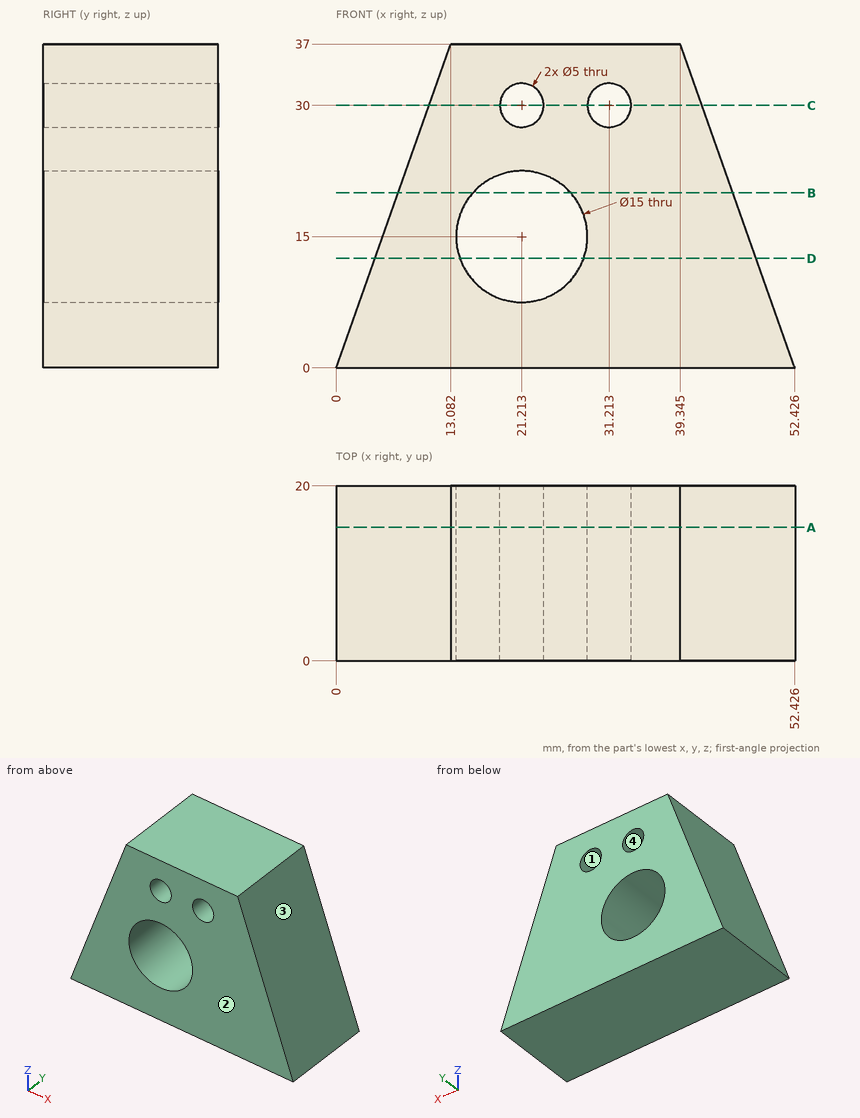
Design review of the part shown in the three views and the two pictorial views. Dimensions are in mm from the part's minimum x, y and z. Give positions to 0.01 mm unless a question says otherwise; leave off trailing zeros. Write each loop counter-clockwise with the first axis right and the second up, starting at its lowest first coordinate (ties: lowest second). Pieces come first, ordered by that corner, then holes. Notation, with made-up numbers: M 11,13 L 68,13 A13 cw 68,24 Z; hole C -25.5,-27.75 d7. An arc over 180 degrees is marked long. Answer in a Markdown table with one row per item.
Item 1: Add section D-D on z = 12.5. Give the boundary of the cut face in (x, y) (1 decimal).
Check sheet entries:
| item | result |
|---|---|
| outline | M 4.4,0 L 14.1,0 L 14.1,20 L 4.4,20 Z; M 28.3,0 L 48,0 L 48,20 L 28.3,20 Z |
Item 2: Draft analysis for pull direction X (two halves, no side actions). For the marked faces 1, 2, 3 and 4, state which applies: +X half, -X half, draft (parallel to the pull), parting line (faces both ways), or undercut.
Check sheet entries:
| item | result |
|---|---|
| face 1 | undercut |
| face 2 | draft |
| face 3 | +X half |
| face 4 | undercut |
Item 3: Add section C-C on z = 30. Give the boundary of the cut face in (x, y), plus the area to 3 significant figures.
Check sheet entries:
| item | result |
|---|---|
| outline | M 10.61,0 L 18.71,0 L 18.71,20 L 10.61,20 Z; M 23.71,0 L 28.71,0 L 28.71,20 L 23.71,20 Z; M 33.71,0 L 41.82,0 L 41.82,20 L 33.71,20 Z |
| area | 424 mm2 |
Item 4: Add section B-B on z = 20. Give the boundary of the cut face in (x, y) (1 decimal), plus the area to 3 significant figures.
Check sheet entries:
| item | result |
|---|---|
| outline | M 7.1,0 L 15.6,0 L 15.6,20 L 7.1,20 Z; M 26.8,0 L 45.4,0 L 45.4,20 L 26.8,20 Z |
| area | 542 mm2 |
Item 5: Add section A-A on y = 15.25. Give the boundary of the cut face in (x, z) (1 decimal), plus the area to 3 significant figures.
Check sheet entries:
| item | result |
|---|---|
| outline | M 0,0 L 52.4,0 L 39.3,37 L 13.1,37 Z; hole C 21.2,15 d15; hole C 21.2,30 d5; hole C 31.2,30 d5 |
| area | 1,240 mm2 |
Item 6: For line 1 along X through (y, z) = (5, 28) (1 decimal); line 2 along Z through (x, y) = (33, 18.5); line 3 along Z through (x, y) = (30.5, 6) (1 decimal), list the stretches that pass through material, from the lowest coordinate up.
Check sheet entries:
| item | result |
|---|---|
| line 1 | 9.9 to 19.7, 22.7 to 29.7, 32.7 to 42.5 |
| line 2 | 0 to 28.25, 31.75 to 37 |
| line 3 | 0 to 27.6, 32.4 to 37 |
Item 7: For P1, Ø1, axis at x = 34, y = 17.5, coming from the -Z side; P2, Ø8, axis at y = 16.5, z = 11.5, coming from the +X side (1 decimal); P3, Ø1.5, axis at y = 3.5, z = 6.5, coming from the -X side, all flat-tipped, find the tip position at first contact; note any pin that passes through.
Check sheet entries:
| item | result |
|---|---|
| P1 | z = 0 |
| P2 | x = 49.8 |
| P3 | x = 2.03 |
